Build history of the part. All positions in model axes, mm. Give positions to 0.01 mm unless a question says otherwise; leave off trailing zeros. Order: outer loops, then holes, each group sorted by start corner. A loop starts at its lowest first (then second) coordinate and runs counter-clockwise, first axis right, second up. Notation, with made-up numbers: (13.5, 83) - (30.5, 83) arc R7 ccw to (30.5, 96) - close; hole circle Ø4 at (78, 47.25). An arc over 180 degrees is marked (long way). Use a Markdown table: item, result. Add a question column.
(1) Flat gauge pins, fed straight in: pin 1 (1.5 mm diameter, centred on y = -105, z = -3.5, fed in from +X); pin 2 (3.5 mm diameter, centred on y = -230, z = 2, fed in from +X); pin 3 (1 mm diameter, centred on y = -144, z = -0.5, fed in from +X) (3 decimals); pin 4 (1.5 mm diameter, centred on y = -79.5, z = 4, fed in from -X). Where does each tip first touch, or does it go through?
(2) Slice it at C-C (z = 2.75). Write the cut outline in (x, y) (3 decimals).
(3) Slice it at A-A (x = 4). Write the cut outline in (y, z) (3 decimals).
(4) Slice it at B-B (y = -312.5). Write the cut outline in (x, z) (3 decimals).
(5) Wall check: line 1 (Y direction, x = 3.5, z = 0.75) (3 decimals); line 2 (X direction, y = -61.5, z = -0.25); line 3 (Z direction, x = 0.5, y = -136). Give the ranges that are in metal, low to high.
from build123d import *

# Parameters (mm, degrees)
F0_R     = 5.715
F1_DEPTH = 457.2
F2_W     = 6.35
F2_H     = 3.175
F3_DEPTH = 5.716


with BuildPart() as f1:
    # F0 (on Front) → F1 (new body)
    with BuildSketch(Plane.XZ):
        Circle(F0_R)
    extrude(amount=F1_DEPTH)

    # F2 (on Top) → F3 (cut, through all)
    with BuildSketch(Plane.XY):
        with Locations((3.175, -230.1875)):
            Rectangle(F2_W, F2_H)
    extrude(amount=F3_DEPTH, mode=Mode.SUBTRACT)


solid = f1.part
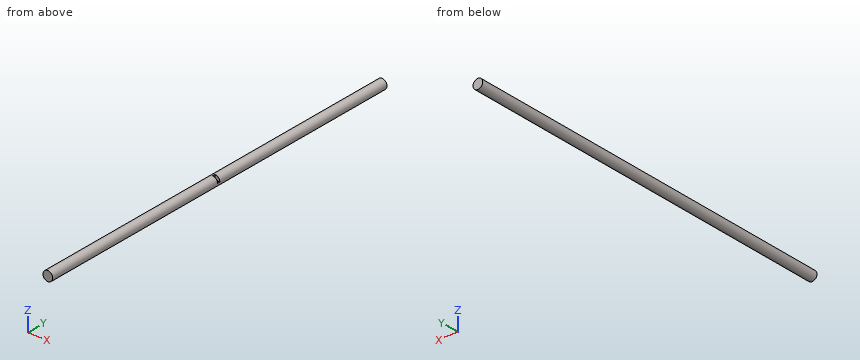
Solution:
| question | item | result |
|---|---|---|
| 1 | pin 1 | x = 5.01 |
| 1 | pin 2 | x = 5.64 |
| 1 | pin 3 | x = 5.715 |
| 1 | pin 4 | x = -4.7 |
| 2 | outline | (-5.01, -457.2) - (5.01, -457.2) - (5.01, -231.775) - (0, -231.775) - (0, -228.6) - (5.01, -228.6) - (5.01, 0) - (-5.01, 0) - close |
| 3 | outline | (-457.2, -4.082) - (0, -4.082) - (0, 4.082) - (-228.6, 4.082) - (-228.6, 0) - (-231.775, 0) - (-231.775, 4.082) - (-457.2, 4.082) - close |
| 4 | outline | circle Ø11.43 at (0, 0) |
| 5 | line 1 | -457.2 to -231.775, -228.6 to 0 |
| 5 | line 2 | -5.71 to 5.71 |
| 5 | line 3 | -5.69 to 5.69 |
